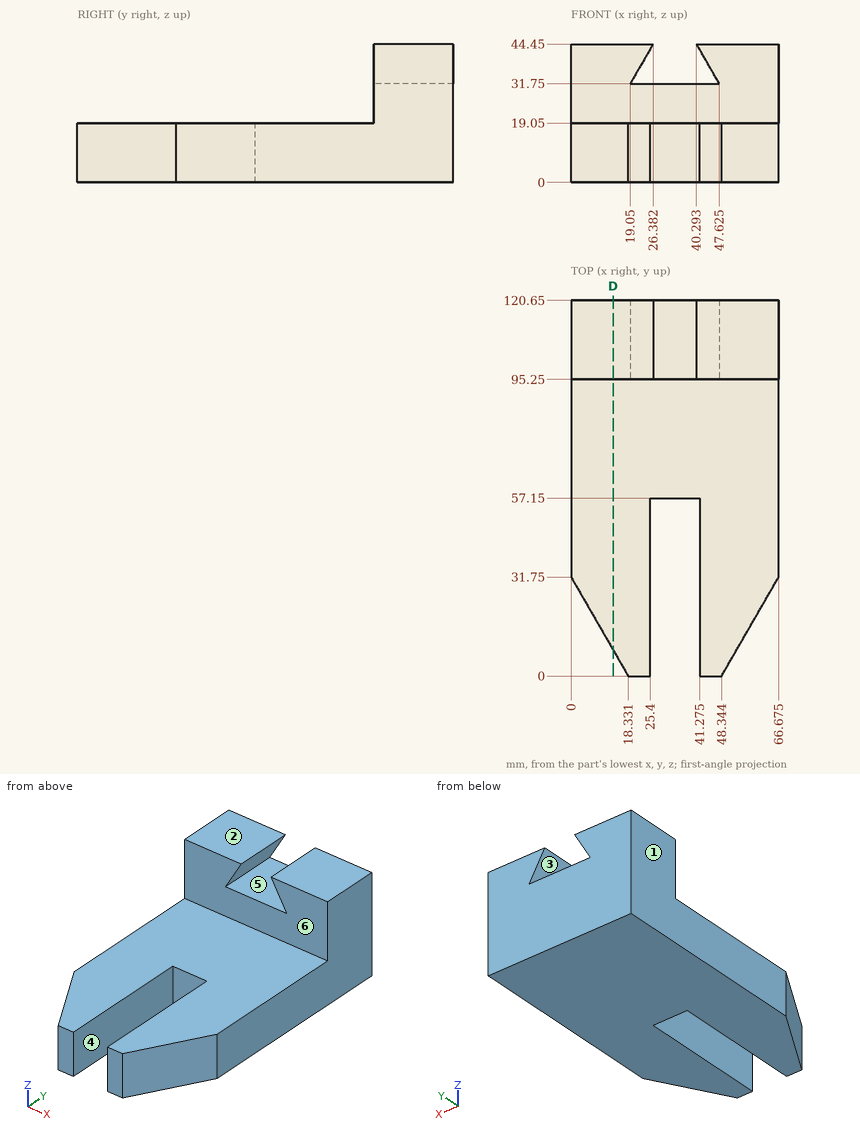
Source: three-view drawing plus pictorial views. Frame: mm from the lowest corner of the part. A direction names the side the tool comes from. Round coordinates to 2 decimals unless told otherwise and drop trailing zeros. Loops run counter-clockwise (first coordinate to the right, second up) from the corner with the lowest first, then second, coordinate; pieces in that order, holes last.
Q1. Pull-direction query (Z, two-part tool) for the marked faces 1, 2 and 3; classes: released by +Z, released by -Z, zero draft, split by the parting line, or undercut.
Q2. Material intervals for L1, parallel to X at y = 54.5, z = 13 (1 decimal); L2, parallel to Y at x = 10, z = 23; L3, parallel to Z at x = 15.5, y = 24.5, sorted ascending.
Q3. Pin query (flat end, axial travel): P1, Ø20, axis at x = 37.5, y = 44.5, coming from the +Z side; P2, Ø4, axis at x = 17, z = 28.5, coming from the -Y side; P3, Ø12.5, axis at x = 34.5, z = 9.5, coming from the -Y side. Return the tip coordinate at first contact, or that it passes through.
Q4. Section D-D on x = 13.5. Return loops of the section in (y, z).
Q5. Access query for the marked faces 4, 5 and 6. Directions: +Z, -Z, +X, -X, +Y, -Y. A direction counts if a zero-diameter tool reaches every point of the face in a straight line with its end or side. Return the directions, or none.
Evaluation:
1. face 1: zero draft
1. face 2: released by +Z
1. face 3: undercut
2. L1: x = 0 to 25.4, 41.3 to 66.7
2. L2: y = 95.25 to 120.65
2. L3: z = 0 to 19.05
3. P1: stops at z = 19.05
3. P2: stops at y = 95.25
3. P3: stops at y = 57.15
4. outline: (8.37, 0) - (120.65, 0) - (120.65, 44.45) - (95.25, 44.45) - (95.25, 19.05) - (8.37, 19.05) - close
5. face 4: +Z, -Z, -Y
5. face 5: +Y, -Y
5. face 6: +Z, +X, -X, -Y
